CAD build for the part. Positions are in the model's coordinates, mm. A direction names the side the tool comes from. Coordinates: 2 decimals unless noted, no trailing zeros. Order: outer loops, then holes, each group sorted by start corner. A loop starts at its lowest first (then second) coordinate and runs counter-clockwise, first axis right, second up.
Autodesk Inventor part; units mm, degrees
ref_plane "YZ Plane" through (0, 0, 0) normal (1, 0, 0) x (0, 1, 0)
ref_plane "XZ Plane" through (0, 0, 0) normal (0, 1, 0) x (-1, 0, 0)
ref_plane "XY Plane" through (0, 0, 0) normal (0, 0, 1) x (1, 0, 0)
sketch "Sketch1" plane through (0, 0, 0) normal (0, 1, 0) x (-1, 0, 0)
  line L0 (0, 0) -> (142.24, 0)
  line L1 (142.24, 0) -> (142.24, -27.94)
  line L2 (142.24, -27.94) -> (0, -27.94)
  line L3 (0, -27.94) -> (0, 0)
  circle A0 centre (76.1968, -16) radius 1.5
  circle A1 centre (56.1968, -16) radius 1.5
  line L4 (146.24, 4) -> (-4, 4)
  line L5 (-4, 4) -> (-4, -31.94)
  line L6 (-4, -31.94) -> (146.24, -31.94)
  line L7 (146.24, -31.94) -> (146.24, 4)
  line L8 (146.24, -6) -> (-4, -6)
  line L9 (-4, -21.94) -> (146.24, -21.94)
  line L10 (127.24, 4) -> (127.24, -31.94)
  line L11 (15, 4) -> (15, -31.94)
  point P0 (127.24, -27.94)
  point P1 (142.24, -21.94)
  point P2 (127.24, 0)
  point P3 (142.24, -6)
  point P4 (15, -27.94)
  point P5 (0, -21.94)
  point P6 (15, 0)
  point P7 (0, -6)
  dimension "d0" = 142.24
  dimension "d1" = 27.94
  dimension "d2" = 3
  dimension "d3" = 3
  dimension "d4" = 20
  dimension "d7" = 16
  dimension "d8" = 4
  dimension "d9" = 4
  dimension "d10" = 4
  dimension "d11" = 4
  dimension "d12" = 15
  dimension "d13" = 15
  dimension "d14" = 10
  dimension "d15" = 10
extrude "Extrusion1" add sketch "Sketch1" along normal blind 5
extrude "Extrusion2" add sketch "Sketch1" along normal blind 30 contours L3 L8 L5 L4 L11 L0 | L10 L4 L7 L8 L1 L0 | L3 L2 L11 L6 L5 L9 | L9 L7 L6 L10 L2 L1
sketch "Sketch2" plane through (0, 5, 0) normal (0, 1, 0) x (1, 0, 0)
  circle A0 centre (-56.1968, 16) radius 1.5
  circle A1 centre (-76.1968, 16) radius 1.5
  line L0 (-146.24, 6) -> (-142.24, 6)
  line L1 (-142.24, 6) -> (-142.24, 0)
  line L2 (-142.24, 0) -> (-127.24, 0)
  line L3 (-127.24, 0) -> (-127.24, -4)
  line L4 (-127.24, -4) -> (-15, -4)
  line L5 (-15, -4) -> (-15, 0)
  line L6 (-15, 0) -> (0, 0)
  line L7 (0, 0) -> (0, 6)
  line L8 (0, 6) -> (4, 6)
  line L9 (4, 6) -> (4, 21.94)
  line L10 (4, 21.94) -> (0, 21.94)
  line L11 (0, 21.94) -> (0, 27.94)
  line L12 (0, 27.94) -> (-15, 27.94)
  line L13 (-15, 27.94) -> (-15, 31.94)
  line L14 (-15, 31.94) -> (-127.24, 31.94)
  line L15 (-127.24, 31.94) -> (-127.24, 27.94)
  line L16 (-127.24, 27.94) -> (-142.24, 27.94)
  line L17 (-142.24, 27.94) -> (-142.24, 21.94)
  line L18 (-142.24, 21.94) -> (-146.24, 21.94)
  line L19 (-146.24, 21.94) -> (-146.24, 6)
  circle A2 centre (-76.1968, 16) radius 3.25
  circle A3 centre (-56.1968, 16) radius 3.25
  dimension "d20" = 6.5
  dimension "d21" = 6.5
extrude "Extrusion3" cut sketch "Sketch2" against normal blind 3.25 contours A0 | A2 | A3
fillet "Fillet1" radius 5 4 edges at (-146.24, 15, -31.94) (-146.24, 15, 4) (4, 15, -31.94) (4, 15, 4)
fillet "Fillet2" radius 2 12 edges at (-144.7755, 30, 2.5355) (-146.24, 30, -3.5) (-134.24, 30, 4) (-144.7755, 30, -30.4755) (-146.24, 30, -24.44) (-134.24, 30, -31.94) (4, 30, -24.44) (-8, 30, -31.94) (2.5355, 30, -30.4755) (-8, 30, 4) (4, 30, -3.5) (2.5355, 30, 2.5355)
fillet "Fillet3" radius 2 26 edges at (-71.12, 5, 4) (-71.12, 5, -31.94) (-127.24, 29.4142, -31.3542) (-127.24, 30, -28.94) (-127.24, 16.5, -31.94) (-127.24, 29.4142, 3.4142) (-127.24, 30, 1) (-127.24, 16.5, 4) (-15, 29.4142, 3.4142) (-15, 30, 1) (-15, 16.5, 4) (-15, 29.4142, -31.3542) (-15, 30, -28.94) (-15, 16.5, -31.94) (3.4142, 29.4142, -6) (1, 30, -6) (4, 16.5, -6) (3.4142, 29.4142, -21.94) (1, 30, -21.94) (4, 16.5, -21.94) (-145.6542, 29.4142, -21.94) (-143.24, 30, -21.94) (-146.24, 16.5, -21.94) (-145.6542, 29.4142, -6) (-143.24, 30, -6) (-146.24, 16.5, -6)
sketch "Sketch3" plane through (0, 5, 0) normal (0, 1, 0) x (1, 0, 0)
  line L0 (-141.24, -4) -> (-1, -4)
  line L1 (-1, 31.94) -> (-141.24, 31.94)
  line L2 (-101.1968, -4) -> (-31.1968, -4)
  line L3 (-31.1968, -4) -> (-31.1968, 31.94)
  line L4 (-31.1968, 31.94) -> (-101.1968, 31.94)
  line L5 (-101.1968, 31.94) -> (-101.1968, -4)
  circle A0 centre (-76.1968, 16) radius 1.5
  circle A1 centre (-56.1968, 16) radius 1.5
  line L6 (-101.1968, 3.5) -> (-31.1968, 3.5)
  line L7 (-31.1968, 3.5) -> (-31.1968, 24.44)
  line L8 (-31.1968, 24.44) -> (-101.1968, 24.44)
  line L9 (-101.1968, 24.44) -> (-101.1968, 3.5)
  point P0 (0, 0)
  point P1 (-31.1968, -4)
  dimension "d27" = 25
  dimension "d28" = 25
  dimension "d29" = 7.5
  dimension "d30" = 7.5
extrude "Extrusion4" cut sketch "Sketch3" against normal blind 18.75 contours L5 L6 L3 L0 | L5 L1 L3 L8
fillet "Fillet4" radius 5 4 edges at (-101.1968, 2.5, -3.5) (-31.1968, 2.5, -3.5) (-31.1968, 2.5, -24.44) (-101.1968, 2.5, -24.44)
properties part number "BatteryHolder"
1) Which spindle directions (+Z, -Z, +X, -X, +Y, -Y) get a long thin tool onto all of the face, cutting with end or side? Do faces 5 (the flat face through (-101.197, 3, 3)), 6 (the flat face through (-58, 1.75, -15)), 7 (the cylindrical face through (-99.693, 2.465, -25.866)). Say none if no direction does.
2) Slice it at A-A (z = -16). List the corners of the cut face in (x, y), plus the area to 3 significant figures.
3) Pin check, flat tips, straight feed: P1, Ø2, axis at x = -76, z = -17.5, coming from the +Y side; P2, Ø4, axis at x = -55.5, z = -19.5, coming from the +Y side; P3, Ø1.6, axis at x = 1, y = 20, coming from the +Z side. Stop position of each tip, or through.
4) Slice it at B-B (x = -135). List the corners of the cut face in (y, z), plus the area to 3 significant figures.
5) Two-plate mould, pull along X, no slides. Class faces 1 (the cylindrical face through (2.57, 14.2, -30.44)), 2 (the flat face through (-75.5, 1.75, -17.5)), 3 (the flat face through (-135, 17, 0)), 4 (the flat face through (-130, 11, 4)): released by +X, released by -X, zero draft, split by the parting line, or undercut.
6) Slice it at D-D (x = -62.5). List the corners of the cut face in (y, z).
7) Slice it at C-C (y = 19.5). Give the number of separate pieces and of enclosed holes in the cut face, plus the area to 3 significant figures.
8) Drill centre lines: probe 1 along X at (y, z) = (2.85, -16); probe 2 along X at (y, z) = (3, -13); probe 3 along Y at (x, z) = (-102.5, -8). Where is each one in solid material? Low to high.
Worked out:
1. face 5: +Z, +Y, -Y
1. face 6: +Y
1. face 7: -Z, +Y, -Y
2. outline: (-146.24, 0) - (-77.7, 0) - (-77.7, 1.75) - (-79.45, 1.75) - (-79.45, 5) - (-146.24, 5) - close; (-74.7, 0) - (-57.7, 0) - (-57.7, 1.75) - (-59.45, 1.75) - (-59.45, 5) - (-72.95, 5) - (-72.95, 1.75) - (-74.7, 1.75) - close; (-54.7, 0) - (4, 0) - (4, 5) - (-52.95, 5) - (-52.95, 1.75) - (-54.7, 1.75) - close
2. area: 698 mm2
3. P1: stops at y = 1.75
3. P2: stops at y = 5
3. P3: stops at z = 3.85
4. outline: (0, -31.94) - (28, -31.94) arc R2 ccw to (30, -29.94) - (30, -27.94) - (5, -27.94) - (5, 0) - (30, 0) - (30, 2) arc R2 ccw to (28, 4) - (0, 4) - close
4. area: 378 mm2
5. face 1: released by +X
5. face 2: undercut
5. face 3: undercut
5. face 4: zero draft
6. outline: (0, -24.44) - (5, -24.44) - (5, -3.5) - (0, -3.5) - close
7. separate pieces: 4
7. enclosed holes: 0
7. area: 372 mm2
8. probe 1: x = -146.24 to -79.45, -72.95 to -59.45, -52.95 to 4
8. probe 2: x = -146.24 to -77.45, -74.95 to -57.45, -54.95 to 4
8. probe 3: y = 0 to 5
